Geometry check sheet. Reference: the model listing, model coordinates, mm. A direction names the side the tool comes from. Round coordinates to 2 decimals unless told otherwise and drop trailing zeros. Order: outer loops, then holes, each group sorted by start corner. A loop starts at its lowest first (then second) coordinate and runs counter-clockwise, first axis right, second up. Notation, with made-up numbers: (-28.5, 84) - (4.5, 84) arc R18 ccw to (4.5, 112) - close; hole circle Ø9 at (29.25, 30.5). An arc over 180 degrees is marked (long way). Return JSON: item names as keys, results as strings. Group by question number.
Q1. Sectioned sample at C-C, the plane y = 14. Record the cut outline in (x, z) (3 decimals).
Q2. Tool access check on faces 4 (the flat face through (-5.57, 27.95, -0.72)), 5 (the flat face through (-5.16, 30.43, -1.03)), 6 (the flat face through (-3.997, 29.919, -1.031)). Record the directions out of +Z, -Z, +X, -X, +Y, -Y that give a thin tool (end or side, any length) a straight path to the whole face; none if there is none.
Q3. Sectioned sample at B-B, the plane x = -11.75. Record the cut outline in (y, z), then the cut area to 3 significant figures.
Q4. Sectioned sample at D-D, the plane y = 3. Record the cut outline in (x, z) (3 decimals), then the cut area to 3 significant figures.
Q5. Gauge pin test, flat ends, axial feed: pin 1 Ø4 at (x, y) = (0.5, 21) entering from +Z (3 decimals); pin 2 Ø1.5 at (y, z) = (25, 3.5) entering from -X; pin 3 Ø3 at (y, z) = (2.5, 6.5) entering from +X; pin 4 Ø7.5 at (x, y) = (-1.5, 16) entering from -Z. Record the tip position at first contact, or that the pin passes through.
Q6. Material ranges on line 1 along Z through (x, y) = (0.5, 5) (3 decimals); line 2 along X through (y, z) = (25, 8.25); line 3 along Z through (x, y) = (-4, 30) (3 decimals), recorded low to high.
Q7. Draft check along Y on faces 1 (the flat face through (-4.221, 31.007, -0.724)), 2 (the flat face through (-1, 14, 3.175)), 3 (the cylindrical face through (-4.642, 30.007, -1.593)). Enter one of: pulls with the +Y half, pulls with the -Y half, needs draft (parallel to the pull), parting line crosses it, or undercut.
Q8. Sectioned sample at A-A, the plane z = 2. Record the cut outline in (x, y), then the cut area to 3 significant figures.
```python
from build123d import *

# Parameters (mm, degrees)
F1_DEPTH  = 3.175
F2_R      = 5.08
F3_R      = 5.08
F5_W      = 3.3427421004
F5_H      = 2.6986296289
F6_DEPTH  = 1.27
F7_R      = 1.27
F8_D      = 1.27
F10_DEPTH = 9.0390737111


with BuildPart() as f1:
    # F0 (on Top) → F1 (new body)
    with BuildSketch(Plane.XY):
        with BuildLine():
            Line((-5.9569855221, 31.7706279457), (-9.597370401, 23.4970282763))
            Line((-9.597370401, 23.4970282763), (-5.4328427644, 21.6646356006))
            Line((-5.4328427644, 21.6646356006), (-4.0882331564, -0.3526416028))
            ThreePointArc((-4.0882331564, -0.3526416028), (0.1973930726, -4.1691933566), (4.0409927589, 0.0921915022))
            Line((4.0409927589, 0.0921915022), (2.6926789221, 27.9647745192))
            Line((2.6926789221, 27.9647745192), (-5.9569855221, 31.7706279457))
        make_face()
    extrude(amount=F1_DEPTH)

    # F2
    f2_edges = [f1.edges().sort_by_distance(p)[0] for p in [
        (2.692679, 27.964775, 1.5875),
    ]]
    fillet(f2_edges, radius=F2_R)

    # F3
    f3_edges = [f1.edges().sort_by_distance(p)[0] for p in [
        (-5.432843, 21.664636, 1.5875),
    ]]
    fillet(f3_edges, radius=F3_R)

    # F5 (on offset) → F6 (join)
    with BuildSketch(Plane(origin=(-15.5400163929, 6.8376091371, 0), x_dir=(-0.4027387092, -0.9153149906, 0), z_dir=(-0.9153149906, 0.4027387092, 0))):
        with Locations((-25.0095250085, -1.3493148144)):
            Rectangle(F5_W, F5_H)
    extrude(amount=-F6_DEPTH)

    # F7
    f7_edges = [f1.edges().sort_by_distance(p)[0] for p in [
        (-4.213362, 31.003294, -2.69863),
        (-5.559613, 27.943632, -2.69863),
    ]]
    fillet(f7_edges, radius=F7_R)

    # F8 (through all)
    with Locations(Plane(origin=(-15.5400163929, 6.8376091371, 0), x_dir=(-0.4027387092, -0.9153149906, 0), z_dir=(-0.9153149906, 0.4027387092, 0))):
        with Locations((-25.0095250085, -1.3493148144)):
            Hole(F8_D / 2)

    # F9 (on face) → F10 (join, through all)
    with BuildSketch(Plane(origin=(10.745480909, 24.4215406479, 0), x_dir=(-0.9153149906, 0.4027387092, 0), z_dir=(0.4027387092, 0.9153149906, 0))):
        Polygon((21.2154332548, 9.9458275363), (18.2477798373, 3.175), (18.2477798373, 0), (19.7086434315, 0), (23.350128904, 8.3082040392), (23.350128904, 9.9458275363), align=None)
    extrude(amount=-F10_DEPTH)


solid = f1.part
```
Reply:
{
 "1": {"outline": "(-4.965, 0) - (3.368, 0) - (3.368, 3.175) - (-4.965, 3.175) - close"},
 "2": {"face 4": "-Z, -X, -Y", "face 5": "-Z, -X, +Y", "face 6": "-Z, +X, -Y"},
 "3": {"outline": "(24.44, 2.03) - (31.27, 8.31) - (31.27, 9.95) - (25.97, 9.95) - (24.44, 8.54) - close", "area": "31.5 mm^2"},
 "4": {"outline": "(-4.293, 0) - (3.9, 0) - (3.9, 3.175) - (-4.293, 3.175) - close", "area": "26.0 mm^2"},
 "5": {"pin 1": "z = 3.175", "pin 2": "x = -12.63", "pin 3": "through", "pin 4": "z = 0"},
 "6": {"line 1": "0 to 3.175", "line 2": "-13.01 to -11.37", "line 3": "-2.621 to 3.175"},
 "7": {"face 1": "pulls with the +Y half", "face 2": "needs draft", "face 3": "undercut"},
 "8": {"outline": "(-11.74, 24.44) - (-8.27, 22.91) arc R5.08 cw to (-5.24, 18.57) - (-4.09, -0.35) arc R4.07 ccw to (4.04, 0.09) - (2.84, 24.83) arc R5.08 ccw to (-0.18, 29.23) - (-8.1, 32.71) - close", "area": "317 mm^2"}
}
